The listing builds one solid part. Answer for the finished solid, in the listing's coordinates (mm). A direction names the side the tool comes from. Give positions to 0.01 mm unless a question says otherwise; leave off trailing zeros. Loops run counter-clockwise (first coordinate to the right, second up) from the corner with the lowest first, then second, coordinate; pieces in that order, holes last. Notation, with made-up numbers: (-34, 69) - (17, 69) arc R9 cw to (17, 73) - close; hole circle Ø10 at (-37.5, -7.75). An arc over 180 degrees is marked (long way). Answer in a Markdown table with one row per item. Add a question column.
```python
from build123d import *

# Parameters (mm, degrees)
SKETCH_4_R          = 9.5
EXTRUDE_1_DEPTH     = 9
SKETCH_5_R          = 5
CUT_EXTRUDE_1_DEPTH = 3.5
SKETCH_6_R          = 8.5
CUT_EXTRUDE_2_DEPTH = 2.5


with BuildPart() as part:
    # 草图4 → 凸台-拉伸1 (new body)
    with BuildSketch(Plane(origin=(0, 0, 0), x_dir=(1, 0, 0), z_dir=(0, 1, 0))):
        Circle(SKETCH_4_R)
    extrude(amount=EXTRUDE_1_DEPTH)

    # 草图5 → 切除-拉伸1 (cut)
    with BuildSketch(Plane(origin=(0, 9, 0), x_dir=(1, 0, 0), z_dir=(0, 1, 0))):
        Circle(SKETCH_5_R)
    extrude(amount=-CUT_EXTRUDE_1_DEPTH, mode=Mode.SUBTRACT)

    # 草图6 → 切除-拉伸2 (cut)
    with BuildSketch(Plane(origin=(0, 5.5, 0), x_dir=(1, 0, 0), z_dir=(0, 1, 0))):
        Circle(SKETCH_6_R)
    extrude(amount=-CUT_EXTRUDE_2_DEPTH, mode=Mode.SUBTRACT)

    # 草图8 → 旋转3 (revolve)
    with BuildSketch(Plane.XY):
        Polygon((9.5, 0), (25, -11), (21.54425858, -11), (6.04425858, 0), align=None)
    revolve(axis=Axis((0, 0, 0), (0, 1, 0)))


solid = part.part
```
(1) The mould has two halves that part along X. Classify faces 4 (the face through (7.3, -11, -20.5)), 5 (the face through (0, 0, 0)), 6 (the face through (4.38, 4.44, 8.43)): pulls with the +X half, pulls with the -X half, needs draft (parallel to the pull), parting line crosses it, or undercut.
(2) A cutting plane is placed at D-D on y = -4.75. Determine the outline of the cut face in (x, z).
(3) A tool of negligible diameter and unlimited length cuts with its end or side. For faces 1 (the face through (-1.08, 7.27, 4.88)), 2 (the face through (4.57, 4.268, -7.167)), 3 (the face through (4, 9, 4)), from which of +Z, -Z, +X, -X, +Y, -Y can it reach the whole face along a straight path? Write none if from no direction.
(4) A cutting plane is placed at B-B on z = 0. Determine the outline of the cut face in (x, y), plus the area to 3 significant figures.
(5) Given pin 1 Ø9.5 at (x, z) = (-3, 2) entering from -Y; pin 2 Ø4 at (x, z) = (3, -12) entering from -Y; pin 3 Ø12 at (y, z) = (4, 11.5) entering from -X, each flat-ended and moving along its own axis, determine where each tip first touches the part or whether it passes through.
(6) A cutting plane is placed at C-C on y = 6.75. Determine the outline of the cut face in (x, z), plus the area to 3 significant figures.
(7) A cutting plane is placed at A-A on x = 0. Determine the outline of the cut face in (y, z).
(8) Find the intervals of material crossed by line 1 along X through (y, z) = (3.75, 0); line 2 along Z through (x, y) = (0, 8), in increasing order. Write a range as [from, to].
Evaluation:
| question | item | result |
|---|---|---|
| 1 | face 4 | needs draft |
| 1 | face 5 | undercut |
| 1 | face 6 | parting line crosses it |
| 2 | outline | circle Ø32.39 at (0, 0); hole circle Ø25.47 at (0, 0) |
| 3 | face 1 | +Y |
| 3 | face 2 | none |
| 3 | face 3 | +Z, -Z, +X, -X, +Y |
| 4 | outline | (-25, -11) - (-21.54, -11) - (-6.04, 0) - (6.04, 0) - (21.54, -11) - (25, -11) - (9.5, 0) - (9.5, 9) - (5, 9) - (5, 5.5) - (8.5, 5.5) - (8.5, 3) - (-8.5, 3) - (-8.5, 5.5) - (-5, 5.5) - (-5, 9) - (-9.5, 9) - (-9.5, 0) - close |
| 4 | area | 170 mm² |
| 5 | pin 1 | stops at y = -1.64 |
| 5 | pin 2 | stops at y = -5.91 |
| 5 | pin 3 | stops at x = -7.75 |
| 6 | outline | circle Ø19 at (0, 0); hole circle Ø10 at (0, 0) |
| 6 | area | 205 mm² |
| 7 | outline | (-11, -25) - (0, -9.5) - (9, -9.5) - (9, -5) - (5.5, -5) - (5.5, -8.5) - (3, -8.5) - (3, 8.5) - (5.5, 8.5) - (5.5, 5) - (9, 5) - (9, 9.5) - (0, 9.5) - (-11, 25) - (-11, 21.54) - (0, 6.04) - (0, -6.04) - (-11, -21.54) - close |
| 8 | line 1 | x = [-9.5, -8.5], [8.5, 9.5] |
| 8 | line 2 | z = [-9.5, -5], [5, 9.5] |
